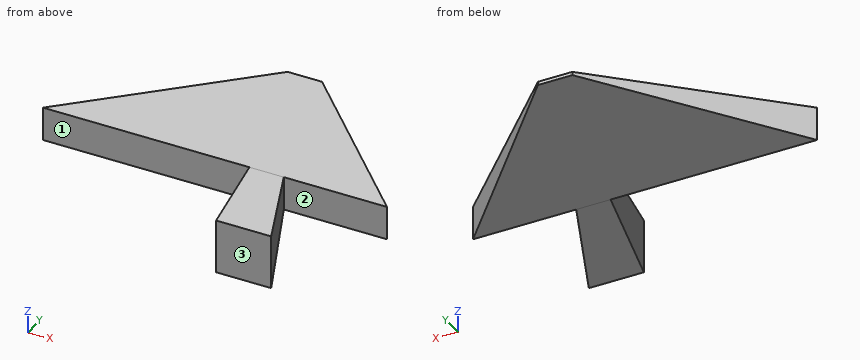
from build123d import *

# Parameters (mm, degrees)
F0_W = 25.4
F0_H = 2.54
F2_W = 254
F2_H = 25.4
F4_W = 25.4
F4_H = 25.4
F6_W = 40.64
F6_H = 40.64


with BuildPart() as f3:
    # F0 (on Front) → F3 section 0
    with BuildSketch(Plane.XZ):
        Rectangle(F0_W, F0_H)
    # F2 (on offset) → F3 section 1
    with BuildSketch(Plane.XZ.offset(127)):
        Rectangle(F2_W, F2_H)
    loft()

    # F4 (on face) → F7 section 0
    with BuildSketch(Plane.XZ.offset(127)):
        with Locations((38.1, 0)):
            Rectangle(F4_W, F4_H)
    # F6 (on offset) → F7 section 1
    with BuildSketch(Plane.XZ.offset(203.2)):
        with Locations((60.96, 0)):
            Rectangle(F6_W, F6_H)
    loft()


solid = f3.part
Geometry: final body of the model. Coordinates: model frame, mm. Face numbers are marked on the shaded views. A direction names the side the tool comes from. Coordinates: 2 decimals unless noted, no trailing zeros. Return JSON: item names as keys, results as strings.
Item 1: Line query: L1, parallel to Y at x = 77, z = -6; L2, parallel to Y at x = -12.5, z = 1; L3, parallel to Z at x = -91.5, y = -98. Output: solid intervals per line, ascending.
Completed:
{"L1": "y = -203.2 to -192.5, -127 to -71.44", "L2": "y = -127 to 0", "L3": "z = -10.09 to 10.09"}
Item 2: Reachability of the marked faces 1, 2 and 3 from +Z, -Z, +X, -X, +Y, -Y: full face, straight path, thin tool, end or side. Return the list, or none.
Completed:
{"face 1": "+Z, -Z, -X, -Y", "face 2": "+Z, -Z, +X", "face 3": "+Z, -Z, +X, -X, -Y"}
Item 3: Pin query (flat end, axial travel): pin 1 Ø10 at (x, y) = (11, -134) entering from -Z; pin 2 Ø6 at (y, z) = (-109.5, 12) entering from +X; pin 3 Ø2 at (x, y) = (-86.5, -91.5) entering from +Z (3 decimals); pin 4 Ø2 at (x, y) = (55.5, -145.5) entering from +Z. Return the tip coordinate at first contact, or that it passes through.
Completed:
{"pin 1": "passes through", "pin 2": "stops at x = 113.89", "pin 3": "stops at z = 9.595", "pin 4": "stops at z = 14.65"}
